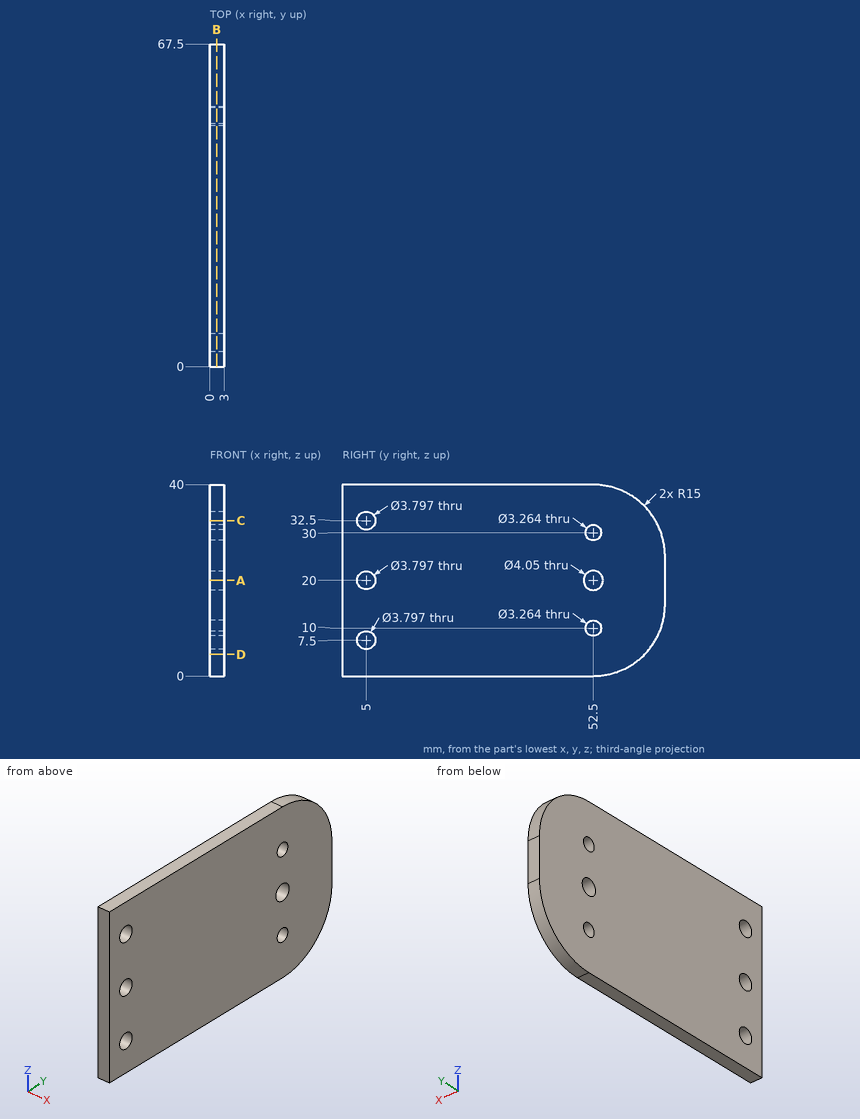
Can you work these out from the drawing? Everything is in mm from the part's minimum corner. Round coordinates to 2 decimals unless told otherwise and drop trailing zeros. Loops run counter-clockwise (first coordinate to the right, second up) from the corner with the lowest first, then second, coordinate; pieces in that order, holes last.
1. If we section it at C-C on z = 32.5: Write out the boundary of the cut face in (x, y).
Answer list:
outline: (0, 0) - (3, 0) - (3, 3.1) - (0, 3.1) - close; (0, 6.9) - (3, 6.9) - (3, 65.49) - (0, 65.49) - close
2. For P1, Ø2.5, axis at y = 5, z = 32.5, coming from the +X side, with a flat end and sliding along its axis, tell me the tip position at first contact or that it passes through.
Answer list:
P1: passes through
3. If I drill on line 1 along Y through (x, z) = (1.7, 20) (1 decimal); line 2 along Z through (x, y) = (1.45, 6) (1 decimal); line 3 along Y through (x, z) = (2.35, 32.5), over which ranges is the centre line in solid material (lowest first)?
Answer list:
line 1: y = 0 to 3.1, 6.9 to 50.5, 54.5 to 67.5
line 2: z = 0 to 5.9, 9.1 to 18.4, 21.6 to 30.9, 34.1 to 40
line 3: y = 0 to 3.1, 6.9 to 65.49
4. If we section it at D-D on z = 4.5: Write out the boundary of the cut face in (x, y), plus the area to 3 significant figures.
Answer list:
outline: (0, 0) - (3, 0) - (3, 63.21) - (0, 63.21) - close
area: 190 mm2
5. If we section it at B-B on x = 1.4: Count the separate pieces of the cut face and the enclosed holes in it, plus the area to 3 significant figures.
Answer list:
separate pieces: 1
enclosed holes: 6
area: 2,540 mm2
6. If we section it at A-A on z = 20: Write out the boundary of the cut face in (x, y) (1 decimal).
Answer list:
outline: (0, 0) - (3, 0) - (3, 3.1) - (0, 3.1) - close; (0, 6.9) - (3, 6.9) - (3, 50.5) - (0, 50.5) - close; (0, 54.5) - (3, 54.5) - (3, 67.5) - (0, 67.5) - close
